Here's how the part is built. I have some questions about the finished solid (model axes, mm). A direction names the side the tool comes from. Coordinates: 2 decimals unless noted, no trailing zeros. Write each loop counter-clockwise with the first axis right and the second up, starting at its lowest first coordinate (ties: lowest second). Pieces come first, ordered by that corner, then holes. Notation, with made-up numbers: (10, 50.5) -> (43, 50.5) arc R28 cw to (43, 86.5) -> close; hole circle Ø4 at (79.5, -8.5). An arc over 180 degrees is marked (long way). Use a Markdown table: item, result. Add a question column.
Item 1: Imagine slicing it at D-D, the plane z = -7.5. Write out the boundary of the cut face in (x, y).
Item 2: If I drill on line 1 along Y through (x, z) = (-7, -0.25); line 2 along Z through (x, y) = (-1, -6.5); line 3 along Z through (x, y) = (-4, -4.75), over which ranges is the centre line in solid material (lowest first)? Write a range as from..to.
Item 3: On a 3-axis mill with a long thin cutter (end or side, diameter ignored), from which of +Z, -Z, +X, -X, +Y, -Y can I reach the whole of each face in a straight line? I mean faces 1 (the cylindrical face through (-0.945, -4.208, 5.925)), 2 (the cylindrical face through (0.932, -4.208, 5.927)), 3 (the cylindrical face through (-4.443, -4.208, -3.242)). Say none if no direction works.
Item 4: Imagine slicing it at B-B, the plane x = 0. Write out the boundary of the cut face in (y, z).
Item 5: Imagine slicing it at A-A, the plane z = 0. Write out the boundary of the cut face in (x, y), and give its area (3 significant figures).
Item 6: Imagine slicing it at C-C, the plane y = -0.75. Write out the boundary of the cut face in (x, z), and give its area (3 significant figures).
Item 7: Will these pins go through, and if not, where does the flat tip stop? pin 1 Ø5 at (y, z) = (-1.5, -6.5) entering from +X; pin 2 Ø1 at (y, z) = (-6, 5) entering from -X; pin 3 Ø3 at (x, y) = (1.5, -6.5) entering from +Z.
Item 8: If we mould it in two halves opening along Y, with no side actions, what happens to faces 4 (the cylindrical face through (-2.44, -4.19, -0.54)), 5 (the flat face through (2, -8.5, 2)), 6 (the flat face through (6, -7.25, 0)), 7 (the cylindrical face through (-5.925, -4.208, -0.945))? For each: pulls with the +Y half, pulls with the -Y half, needs draft (parallel to the pull), parting line crosses it, or undercut.
```python
from build123d import *

# Parameters (mm, degrees)
SKETCH_2_R               = 2.5
CUT_EXTRUDE_1_DEPTH      = 10
SKETCH_5_R               = 0.5
CUT_EXTRUDE_3_DEPTH      = 6
PATTERN_CIRCULAR_2_COUNT = 20


with BuildPart() as part:
    # 草图1 → 旋转1 (revolve)
    with BuildSketch(Plane.XY, mode=Mode.PRIVATE) as revolve_1_sk:
        Polygon((0, -8.5), (-9, -8.5), (-9, -7.25), (-6, -7.25), (-6, -1.25), (-9, -1.25), (-9, 0), (0, 0), align=None)
    revolve(revolve_1_sk.sketch.rotate(Axis((0, 0, 0), (0, 1, 0)), 270), axis=Axis((0, 0, 0), (0, 1, 0)))

    # 草图2 → 切除-拉伸1 (cut)
    with BuildSketch(Plane(origin=(0, 0, 0), x_dir=(1, 0, 0), z_dir=(0, 1, 0))):
        with Locations(Location((0, 0, 0), (0, 0, 270))):
            Circle(SKETCH_2_R)
    extrude(amount=-CUT_EXTRUDE_1_DEPTH, mode=Mode.SUBTRACT)

    # 草图5 → 切除-拉伸3 (cut)
    with BuildSketch(Plane.XZ.offset(1.25)):
        with Locations((0, 6)):
            Circle(SKETCH_5_R)
    cut_extrude_3 = extrude(amount=CUT_EXTRUDE_3_DEPTH, mode=Mode.SUBTRACT)

    # 阵列(圆周)2: 切除-拉伸3 ×20 about axis
    pattern_circular_2_axis = Axis((0, 0, 0), (0, 1, 0))
    for i in range(1, PATTERN_CIRCULAR_2_COUNT):
        add(cut_extrude_3.rotate(pattern_circular_2_axis, i * 360 / PATTERN_CIRCULAR_2_COUNT), mode=Mode.SUBTRACT)


solid = part.part
```
Ans:
| question | item | result |
|---|---|---|
| 1 | outline | (-4.97, -8.5) -> (4.97, -8.5) -> (4.97, -7.25) -> (-4.97, -7.25) -> close; (-4.97, -1.25) -> (4.97, -1.25) -> (4.97, 0) -> (-4.97, 0) -> close |
| 2 | line 1 | y = -8.5..-7.25, -1.25..0 |
| 2 | line 2 | z = -5.92..-2.29, 2.29..5.92 |
| 2 | line 3 | z = -4.47..4.47 |
| 3 | face 1 | +Z, -X |
| 3 | face 2 | +Z, +X |
| 3 | face 3 | none |
| 4 | outline | (-8.5, -9) -> (-7.25, -9) -> (-7.25, -5.5) -> (-1.25, -5.5) -> (-1.25, -9) -> (0, -9) -> (0, -2.5) -> (-8.5, -2.5) -> close; (-8.5, 2.5) -> (0, 2.5) -> (0, 9) -> (-1.25, 9) -> (-1.25, 5.5) -> (-7.25, 5.5) -> (-7.25, 9) -> (-8.5, 9) -> close |
| 5 | outline | (-9, -8.5) -> (-2.5, -8.5) -> (-2.5, 0) -> (-9, 0) -> (-9, -1.25) -> (-5.5, -1.25) -> (-5.5, -7.25) -> (-9, -7.25) -> close; (2.5, -8.5) -> (9, -8.5) -> (9, -7.25) -> (5.5, -7.25) -> (5.5, -1.25) -> (9, -1.25) -> (9, 0) -> (2.5, 0) -> close |
| 5 | area | 68.5 mm^2 |
| 6 | outline | circle Ø18 at (0, 0); hole circle Ø5 at (0, 0) |
| 6 | area | 235 mm^2 |
| 7 | pin 1 | stops at x = 8.06 |
| 7 | pin 2 | stops at x = -3.97 |
| 7 | pin 3 | stops at z = 9 |
| 8 | face 4 | needs draft |
| 8 | face 5 | pulls with the -Y half |
| 8 | face 6 | undercut |
| 8 | face 7 | undercut |
